```python
from build123d import *

# Parameters (mm, degrees)
CYLINDER001_R     = 4.02
CYLINDER001_DEPTH = 2.51
CYLINDER_R        = 5.1
CYLINDER_DEPTH    = 3.5
FILLET_R          = 0.5


with BuildPart() as cylinder001:
    # Cylinder001 → Cylinder001 (new body)
    with BuildSketch(Plane.XY):
        Circle(CYLINDER001_R)
    extrude(amount=CYLINDER001_DEPTH)


with BuildPart() as fillet_body:
    # Cylinder → Cylinder (new body)
    with BuildSketch(Plane.XY):
        Circle(CYLINDER_R)
    extrude(amount=CYLINDER_DEPTH)

    # Cut: cut Cylinder001
    add(cylinder001.part, mode=Mode.SUBTRACT)

    # Fillet
    fillet_edges = [fillet_body.edges().sort_by_distance(p)[0] for p in [
        (-5.1, 0, 3.5),
    ]]
    fillet(fillet_edges, radius=FILLET_R)


solid = fillet_body.part
```
Source: CAD feature listing. Evaluate the final solid. Frame: model axes, mm. A direction names the side the tool comes from. Coordinates: 2 decimals unless noted, no trailing zeros. Order: outer loops, then holes, each group sorted by start corner. A loop starts at its lowest first (then second) coordinate and runs counter-clockwise, first axis right, second up. Notation, with made-up numbers: M 60,-33.75 L 84,-33.75 A6 cw 84,-22.75 Z; hole C 24.5,60.5 d1. An arc over 180 degrees is marked long. Write each question's results on one line, items separated by ' | '. Start each with the question number.
1) Contact query for flat-ended pins moving along their axis: pin 1 Ø1 at (x, y) = (-1, 1.5) entering from -Z; pin 2 Ø2 at (x, z) = (2, 3) entering from +Y. Output: stop coordinate, or through.
2) Access query for faces 1 (the face through (4, 2, 0)), 2 (the face through (0, 0, 2.51)). Directions: +Z, -Z, +X, -X, +Y, -Y. A direction counts if a zero-diameter tool reaches every point of the face in a straight line with its end or side. Return the directions, or none.
3) Draft query along X for faces 3 (the face through (3.834, 1.207, 1.237)), 4 (the face through (0, 0, 3.5)), 5 (the face through (2.4, -4.5, 1.5)). Return one class per face: released by +X, released by -X, zero draft, split by the parting line, or undercut.
4) Section query A-A (y = 0). Return the cut outline in (x, z), plus the area to 3 significant figures.
5) Line query: line 1 (Y direction, x = 0, z = 1.5); line 2 (Z direction, x = 0, y = 0); line 3 (X direction, y = -3.25, z = 1). Output: solid intervals per line, ascending. Write a range as from..to.
6) Section query C-C (z = 0.3). Return the cut outline in (x, y), plus the area to 3 significant figures.
7) Section query D-D (z = 2.7). Return the cut outline in (x, y).
Answers:
1) pin 1: stops at z = 2.51 | pin 2: stops at y = 5
2) face 1: -Z, +X, -X, +Y, -Y | face 2: -Z
3) face 3: undercut | face 4: zero draft | face 5: split by the parting line
4) outline: M -5.1,0 L -4.02,0 L -4.02,2.51 L 4.02,2.51 L 4.02,0 L 5.1,0 L 5.1,3 A0.5 ccw 4.6,3.5 L -4.6,3.5 A0.5 ccw -5.1,3 Z | area: 15.4 mm^2
5) line 1: y = -5.1..-4.02, 4.02..5.1 | line 2: z = 2.51..3.5 | line 3: x = -3.93..-2.37, 2.37..3.93
6) outline: C 0,0 d10.2; hole C 0,0 d8.04 | area: 30.9 mm^2
7) outline: C 0,0 d10.2
